CAD build for the part. Positions are in the model's coordinates, mm. Coordinates: 2 decimals unless noted, no trailing zeros. Loops run counter-clockwise (first coordinate to the right, second up) from the corner with the lowest first, then second, coordinate; pieces in that order, holes last. Notation, with made-up numbers: (20, 30.25) -> (62, 30.25) arc R26 cw to (62, 56.25) -> close; hole circle Ø4 at (-13.75, 62). An arc over 180 degrees is marked (long way). Return JSON: item names as keys, results as strings. Group by question number.
(1) Saw through at B-B on x = 134.5. Write the cut outline in (y, z), then the cut area to 3 significant figures.
(2) Saw through at A-A on y = 0. Write the cut outline in (x, z).
(3) Probe L1, parallel to X at y = 1, z = 1.4; L2, parallel to X at y = 1.5, z = 2.5; L3, parallel to Y at x = 134.5, z = 1.8. List the from-to ranges inside material, lowest first.
(4) Flat gauge pin, fed straight in: pin 1 Ø1 at (y, z) = (1.5, 2.5) entering from +X. Where does the tip first touch, or does it go through?
(5) Saw through at D-D on x = 154.5. Write the cut outline in (y, z).
(6) Saw through at C-C on z = 1.25. Write the cut outline in (x, y), then the cut area to 3 significant figures.
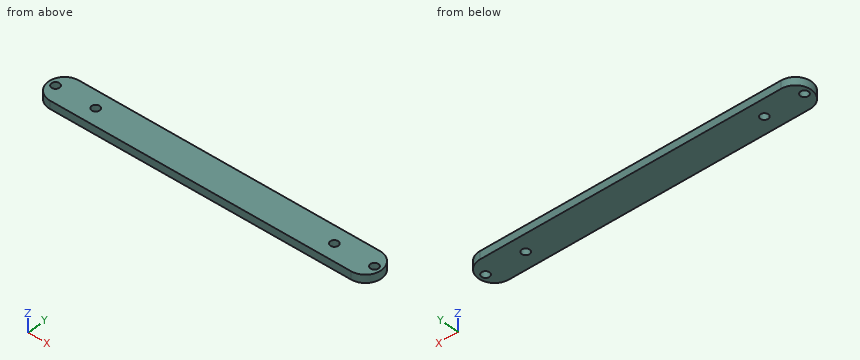
```python
from build123d import *

# Parameters (mm, degrees)
EXTRUDE_1_DEPTH     = 4
SKETCH_2_R          = 2
CUT_EXTRUDE_1_DEPTH = 10


with BuildPart() as part:
    # 草图1 → 凸台-拉伸1 (new body)
    with BuildSketch(Plane.XY):
        with BuildLine():
            Line((0, 8), (150, 8))
            ThreePointArc((150, 8), (158, 0), (150, -8))
            Line((150, -8), (0, -8))
            ThreePointArc((0, -8), (-8, 0), (0, 8))
        make_face()
    extrude(amount=EXTRUDE_1_DEPTH)

    # 草图2 → 切除-拉伸1 (cut)
    with BuildSketch(Plane.XY.offset(4)):
        with Locations((15.5, 0)):
            Circle(SKETCH_2_R)
        with Locations((134.5, 0)):
            Circle(SKETCH_2_R)
        with Locations((-4.5, 0)):
            Circle(SKETCH_2_R)
        with Locations((154.5, 0)):
            Circle(SKETCH_2_R)
    extrude(amount=-CUT_EXTRUDE_1_DEPTH, mode=Mode.SUBTRACT)


solid = part.part
```
Geometry results:
{
 "1": {"outline": "(-8, 0) -> (-2, 0) -> (-2, 4) -> (-8, 4) -> close; (2, 0) -> (8, 0) -> (8, 4) -> (2, 4) -> close", "area": "48.0 mm²"},
 "2": {"outline": "(-8, 0) -> (-6.5, 0) -> (-6.5, 4) -> (-8, 4) -> close; (-2.5, 0) -> (13.5, 0) -> (13.5, 4) -> (-2.5, 4) -> close; (17.5, 0) -> (132.5, 0) -> (132.5, 4) -> (17.5, 4) -> close; (136.5, 0) -> (152.5, 0) -> (152.5, 4) -> (136.5, 4) -> close; (156.5, 0) -> (158, 0) -> (158, 4) -> (156.5, 4) -> close"},
 "3": {"L1": "-7.94 to -6.23, -2.77 to 13.77, 17.23 to 132.77, 136.23 to 152.77, 156.23 to 157.94", "L2": "-7.86 to -5.82, -3.18 to 14.18, 16.82 to 133.18, 135.82 to 153.18, 155.82 to 157.86", "L3": "-8 to -2, 2 to 8"},
 "4": {"pin 1": "x = 157.94"},
 "5": {"outline": "(-6.61, 0) -> (-2, 0) -> (-2, 4) -> (-6.61, 4) -> close; (2, 0) -> (6.61, 0) -> (6.61, 4) -> (2, 4) -> close"},
 "6": {"outline": "(0, -8) -> (150, -8) arc R8 ccw to (150, 8) -> (0, 8) arc R8 ccw to start; hole circle Ø4 at (-4.5, 0); hole circle Ø4 at (15.5, 0); hole circle Ø4 at (134.5, 0); hole circle Ø4 at (154.5, 0)", "area": "2,550 mm²"}
}
